Source: three-view drawing plus pictorial views. Frame: mm from the lowest corner of the part. A direction names the side the tool comes from. Give positions to 0.01 mm unless a question says otherwise; leave off trailing zeros. Write each loop counter-clockwise with the first axis right and the second up, starting at its lowest first coordinate (ties: lowest second). Pieces come first, ordered by that corner, then holes.
Q1. Cut plane A-A on z = 4.5. Return the cut outline in (x, y), plus the area to 3 significant figures.
Q2. Pin query (flat end, axial travel): pin 1 (1.5 mm diameter, centred on x = 3, z = 2.5, fed in from -Y). Return the tip coordinate at first contact, or that it passes through.
Q3. Cut plane D-D on x = 3. Return the cut outline in (y, z), plus the area to 3 significant figures.
Q4. Line query: L1, parallel to Y at x = 0.6, z = 4.5; L2, parallel to Z at x = 0.75, y = 4.5; L3, parallel to X at y = 17, z = 2.5. Output: solid intervals per line, ascending.
Q5. Reachability of the marked faces 1 and 2 from +Z, -Z, +X, -X, +Y, -Y: full face, straight path, thin tool, end or side. Return the list, or none.
Q6. Cut plane B-B on y = 2. Return the cut outline in (x, z), plus the area to 3 significant figures.
Q7. Draft query along X for the marked faces 3, 4, 5 and 6. Return one class per face: pulls with the +X half, pulls with the -X half, needs draft (parallel to the pull), parting line crosses it, or undercut.
Q8. Cut plane C-C on y = 22.5. Return the cut outline in (x, z), plus the area to 3 significant figures.
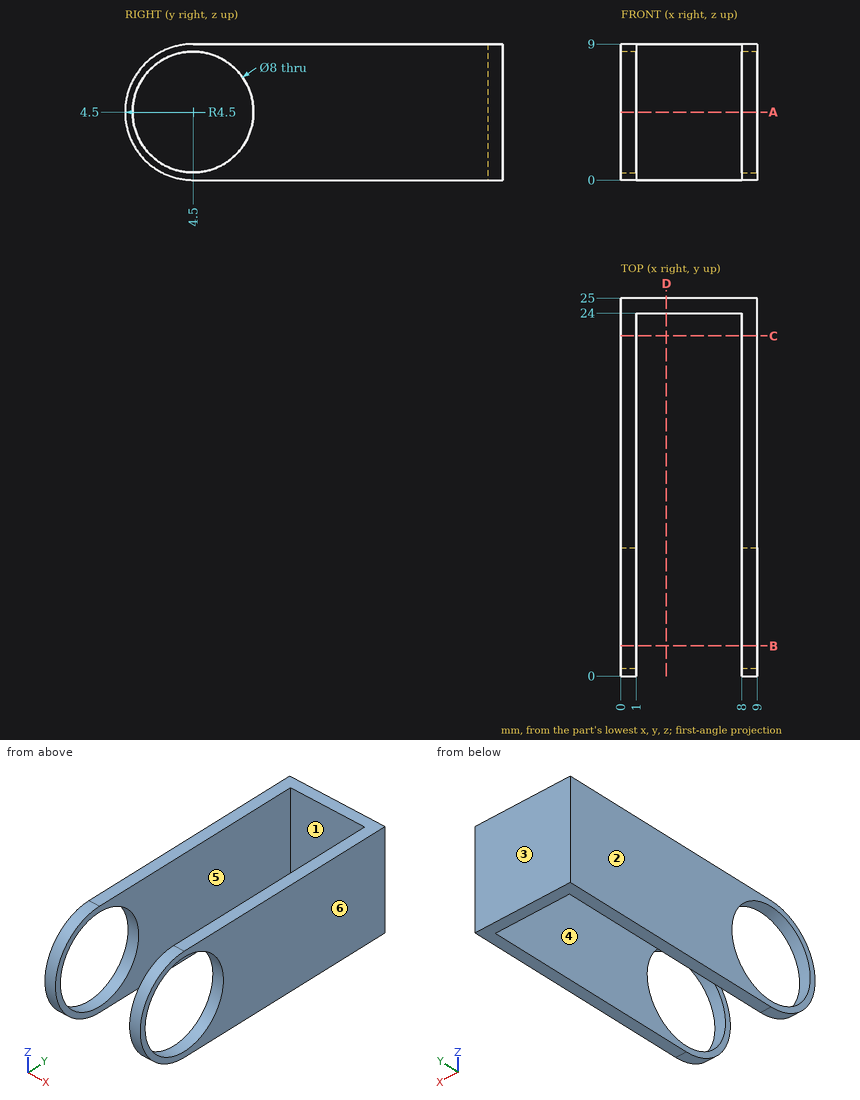
Data:
1. outline: (0, 0) - (1, 0) - (1, 0.5) - (0, 0.5) - close; (0, 8.5) - (1, 8.5) - (1, 24) - (8, 24) - (8, 8.5) - (9, 8.5) - (9, 25) - (0, 25) - close; (8, 0) - (9, 0) - (9, 0.5) - (8, 0.5) - close
1. area: 41.0 mm2
2. pin 1: stops at y = 24
3. outline: (24, 0) - (25, 0) - (25, 9) - (24, 9) - close
3. area: 9.00 mm2
4. L1: y = 0 to 0.5, 8.5 to 25
4. L2: z = 0 to 0.5, 8.5 to 9
4. L3: x = 0 to 1, 8 to 9
5. face 1: +Z, -Z, -Y
5. face 2: +Z, -Z, -X, +Y, -Y
6. outline: (0, 0.76) - (1, 0.76) - (1, 1.38) - (0, 1.38) - close; (0, 7.62) - (1, 7.62) - (1, 8.24) - (0, 8.24) - close; (8, 0.76) - (9, 0.76) - (9, 1.38) - (8, 1.38) - close; (8, 7.62) - (9, 7.62) - (9, 8.24) - (8, 8.24) - close
6. area: 2.48 mm2
7. face 3: needs draft
7. face 4: undercut
7. face 5: undercut
7. face 6: pulls with the +X half
8. outline: (0, 0) - (1, 0) - (1, 9) - (0, 9) - close; (8, 0) - (9, 0) - (9, 9) - (8, 9) - close
8. area: 18.0 mm2
